```python
from build123d import *

# Parameters (mm, degrees)
F0_W      = 8.3
F0_H      = 10.8
F1_ANGLE  = 45
F2_W      = 8
F2_H      = 10.5
F3_DEPTH  = 10
F4_R      = 5.24999
F5_R      = 3.5
F6_DEPTH  = 17.0010001
F7_DEPTH  = 10.15
F8_R      = 5.39999
F9_W      = 20
F9_H      = 70
F10_DEPTH = 50
F11_R     = 3.35
F11_R_2   = 1.65
F12_DEPTH = 4.15
F13_DEPTH = 25
F14_R     = 1.65
F15_DEPTH = 25
F16_DEPTH = 5.5
F17_R     = 0.5


# Not quite as in the source:
# - a fillet or chamfer is up to 0.001 mm smaller than in the source, because OpenCascade refuses the exact size


with BuildPart() as f1:
    # F0 (on Top) → F1 (revolve)
    with BuildSketch(Plane.XY):
        with BuildLine():
            add(Edge.make_bspline(
                [(0, 14), (-22.5166604984, 14), (-11.2583302492, -7), (0, -28), (11.2583302492, -7), (22.5166604984, 14), (0, 14)],
                knots=[0, 0, 0, 2.0943951024, 2.0943951024, 4.1887902048, 4.1887902048, 6.2831853072, 6.2831853072, 6.2831853072], degree=2, weights=[1, 0.5, 1, 0.5, 1, 0.5, 1]))
        make_face()
        Rectangle(F0_W, F0_H, mode=Mode.SUBTRACT)
        Rectangle(F0_W, F0_H)
    revolve(axis=Axis((13.7635422871, 50, 0), (-1, 0, 0)), revolution_arc=F1_ANGLE)

    # F2 (on face) → F3 (join)
    with BuildSketch(Plane(origin=(0, 25, 25), x_dir=(1, 0, 0), z_dir=(0, 0.7071067812, 0.7071067812))):
        with Locations((0, -14.6446609407)):
            Rectangle(F2_W, F2_H)
    extrude(amount=F3_DEPTH)

    # F4 (radius 5.25 in the source; OpenCascade refuses exactly that, so slightly less here)
    f4_edges = [f1.edges().sort_by_distance(p)[0] for p in [
        (0, 18.003418, 46.138717),
        (0, 25.428039, 38.714096),
    ]]
    fillet(f4_edges, radius=F4_R)

    # F5 (on face) → F6 (cut, through all)
    with BuildSketch(Plane.YZ.offset(4)):
        with Locations((18.0034181513, 38.71409627)):
            Circle(F5_R)
    extrude(amount=-F6_DEPTH, mode=Mode.SUBTRACT)

    # F0 (on Top) → F7 (cut)
    with BuildSketch(Plane.XY):
        Rectangle(F0_W, F0_H)
    extrude(amount=F7_DEPTH, mode=Mode.SUBTRACT)

    # F8 (radius 5.4 in the source; OpenCascade refuses exactly that, so slightly less here)
    f8_edges = [f1.edges().sort_by_distance(p)[0] for p in [
        (0, 5.4, 10.15),
        (0, -5.4, 10.15),
    ]]
    fillet(f8_edges, radius=F8_R)

    # F9 (on Top) → F10 (intersect)
    with BuildSketch(Plane.XY):
        with Locations((10, 0)):
            Rectangle(F9_W, F9_H)
    extrude(amount=F10_DEPTH, mode=Mode.INTERSECT)

    # F11 (on face) → F12 (join)
    with BuildSketch(Plane(origin=(4.15, 0, 0), x_dir=(0, -1, 0), z_dir=(-1, 0, 0))):
        with Locations((0, 4.75)):
            Circle(F11_R)
        with Locations((0, 4.75)):
            Circle(F11_R_2, mode=Mode.SUBTRACT)
    extrude(amount=F12_DEPTH)

    # F13 (cut): a face of the model
    f13_faces = [f1.faces().sort_by_distance(p)[0] for p in [
        (4.15, 0, 4.75),
    ]]
    extrude(f13_faces, amount=-F13_DEPTH, mode=Mode.SUBTRACT)

    # F14 (on face) → F15 (cut)
    with BuildSketch(Plane(origin=(4.15, 0, 0), x_dir=(0, -1, 0), z_dir=(-1, 0, 0))):
        Polygon((1.6454482672, 7.6), (-1.6454482672, 7.6), (-3.2908965344, 4.75), (-1.6454482672, 1.9), (1.6454482672, 1.9), (3.2908965344, 4.75), align=None)
        with Locations((0, 4.75)):
            Circle(F14_R, mode=Mode.SUBTRACT)
    extrude(amount=-F15_DEPTH, mode=Mode.SUBTRACT)

    # F14 (on face) → F16 (join)
    with BuildSketch(Plane(origin=(4.15, 0, 0), x_dir=(0, -1, 0), z_dir=(-1, 0, 0))):
        Polygon((1.6454482672, 7.6), (-1.6454482672, 7.6), (-3.2908965344, 4.75), (-1.6454482672, 1.9), (1.6454482672, 1.9), (3.2908965344, 4.75), align=None)
        with Locations((0, 4.75)):
            Circle(F14_R, mode=Mode.SUBTRACT)
    extrude(amount=-F16_DEPTH)

    # F17
    f17_edges = [f1.edges().sort_by_distance(p)[0] for p in [
        (12.999956, -0.000217, 1.9),
        (12.77819, -2.469724, 3.327687),
        (12.731462, -2.468902, 6.173737),
        (12.988931, -0.003353, 7.6),
        (12.857066, 2.469489, 6.17272),
        (12.81516, 2.468662, 3.325848),
        (9.65, 1.65, 4.75),
    ]]
    fillet(f17_edges, radius=F17_R)


solid = f1.part
```
Input: part model. Units: mm. Frame: model coordinates. A direction names the side the tool comes from. Coordinates: 2 decimals unless noted, no trailing zeros. Use a Markdown table: item, result. Add a question column.
1) Draft query along Z for faces 1 (the flat face through (0, 2, 4)), 2 (the flat face through (11, 0, 1.9)), 3 (the cylindrical face through (2.028, 17.946, 43.964)). Return one class per face: +Z half, -Z half, draft (parallel to the pull), parting line (faces both ways), or undercut.
2) Pin query (flat end, axial travel): P1, Ø5, axis at x = 9, z = 35, coming from the +Y side; P2, Ø10, axis at y = 20, z = 35.5, coming from the +X side; P3, Ø8, axis at y = 17, z = 26, coming from the +X side. Return the tip coordinate at first contact, or that it passes through.
3) Line query: L1, parallel to Z at x = 1.5, y = 0; L2, parallel to Z at x = 3.25, y = 21; L3, parallel to Z at x = 8.05, y = 0. Output: solid intervals per line, ascending. Write a range as from..to.
4) Set-up query: faces 4 (the flat face through (6, 15, 35)), 5 (the flat face through (1.972, 20.013, 33.299)), 6 (the cylindrical face through (2.104, -3.86, 8.526)). Return all of +Z, -Z, +X, -X, +Y, -Y with unobstructed straight access to the full face (end or side cutting, diameter ignored); none if empty.
Answer below:
| question | item | result |
|---|---|---|
| 1 | face 1 | draft |
| 1 | face 2 | undercut |
| 1 | face 3 | +Z half |
| 2 | P1 | y = 17.5 |
| 2 | P2 | x = 12.99 |
| 2 | P3 | x = 12.46 |
| 3 | L1 | 1.4..3.1, 6.4..8.1, 10.15..39.8 |
| 3 | L2 | 22.07..29, 34.29..36.91, 40.52..43.02 |
| 3 | L3 | 0..3.1, 6.4..34.93 |
| 4 | face 4 | +X |
| 4 | face 5 | +X, -X, +Y |
| 4 | face 6 | -X |
